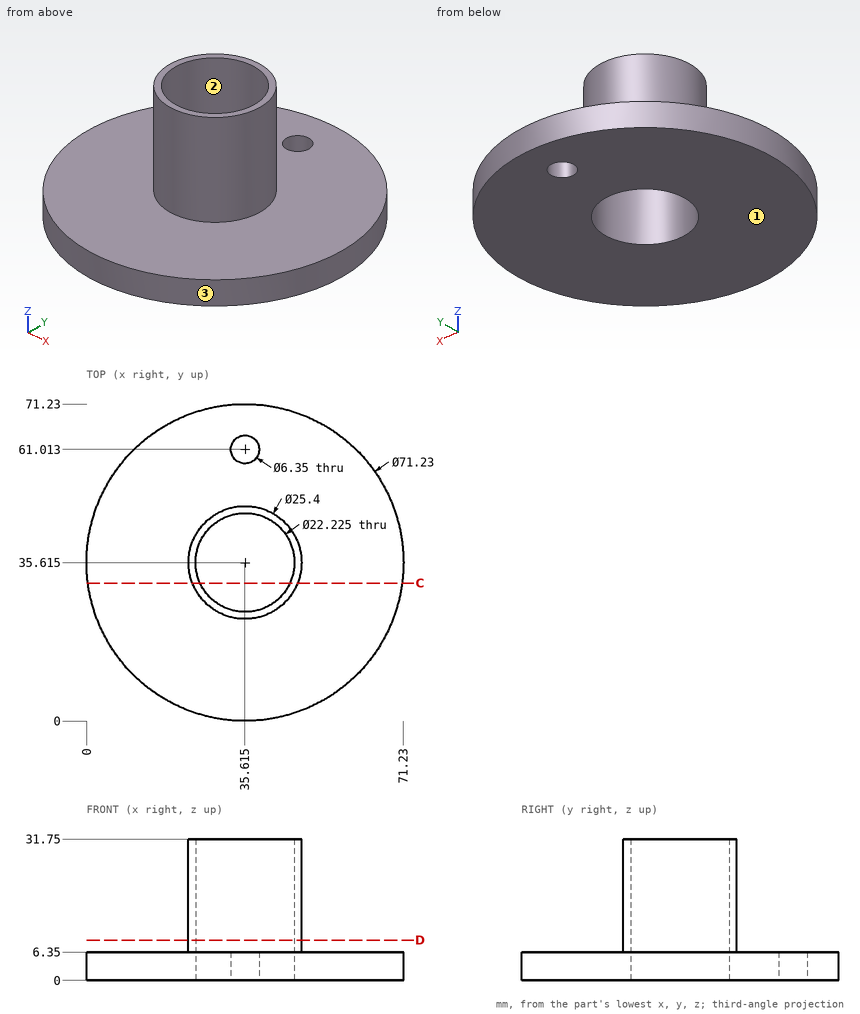
Source: three-view drawing plus pictorial views. Frame: mm from the lowest corner of the part. Give positions to 0.01 mm unless a question says otherwise; leave off trailing zeros. Order: outer loops, then holes, each group sorted by start corner. A loop starts at its lowest first (then second) coordinate and runs counter-clockwise, first axis right, second up. Notation, with made-up numbers: M -27.5,57.25 L -23.5,57.25 A19 cw -23.5,93.25 Z; hole C 70.5,65.25 d8. An arc over 180 degrees is marked long. Return JSON: item names as keys, results as strings.
1) Line query: L1, parallel to X at y = 36, z = 16.5; L2, parallel to Z at x = 23, y = 52; L3, parallel to X at y = 27.5, z = 13 (1 decimal). Output: solid intervals per line, ascending. Write a range as [from, to].
Taken from the geometry:
{"L1": "x = [22.92, 24.51], [46.72, 48.31]", "L2": "z = [0, 6.35]", "L3": "x = [25.8, 28], [43.2, 45.4]"}
2) Contact query for flat-ended pins moving along their axis: pin 1 (3 mm diameter, centred on x = 44.5, y = 32.5, fed in from +Z); pin 2 (3 mm diameter, centred on x = 30, z = 12.5, fed in from -Y); pin 3 (8 mm diameter, centred on x = 22.5, z = 28.5, fed in from +Y); pin 4 (12 mm diameter, centred on y = 27, z = 28.5, fed in from -X). Output: stop coordinate, or through.
Taken from the geometry:
{"pin 1": "passes through", "pin 2": "stops at y = 23.6", "pin 3": "stops at y = 44.46", "pin 4": "stops at x = 23.19"}
3) Section query C-C on y = 31. Output: boundary loops of the cut face in (x, z).
Taken from the geometry:
{"outline": "M 0.3,0 L 25.51,0 L 25.51,31.75 L 23.78,31.75 L 23.78,6.35 L 0.3,6.35 Z; M 45.72,0 L 70.93,0 L 70.93,6.35 L 47.45,6.35 L 47.45,31.75 L 45.72,31.75 Z"}
4) Section query D-D on z = 9. Output: boundary loops of the cut face in (x, y) (1 decimal).
Taken from the geometry:
{"outline": "C 35.6,35.6 d25.4; hole C 35.6,35.6 d22.2"}
5) Mould query, pull axis X, two halves, no side actions, for the marked faces 1, 2 and 3. Classes: released by +X, released by -X, zero draft, split by the parting line, or undercut.
Taken from the geometry:
{"face 1": "zero draft", "face 2": "undercut", "face 3": "split by the parting line"}
